```python
from build123d import *

# Parameters (mm, degrees)
HIERRO_ANGULAR_2_X_2_X_0_125_1_DEPTH = 120
CROQUIS3_W                           = 47.625
CROQUIS3_H                           = 45
CORTAR_EXTRUIR1_DEPTH                = 10
CROQUIS4_R                           = 5
CROQUIS4_R_2                         = 2.5
CORTAR_EXTRUIR2_DEPTH                = 10
CROQUIS5_R                           = 16
CORTAR_EXTRUIR3_DEPTH                = 3.175
CROQUIS6_R                           = 2
CORTAR_EXTRUIR4_DEPTH                = 3.175


with BuildPart() as part:
    # Sketch1 → Hierro angular 2 X 2 X 0.125(1) (new body)
    with BuildSketch(Plane(origin=(0, 0, 0), x_dir=(-1, 0, 0), z_dir=(0, 1, 0))):
        with BuildLine():
            Line((0, 0), (0, 50.8))
            Line((0, 50.8), (0.00508, 50.8))
            ThreePointArc((0.00508, 50.8), (2.246551928, 49.871551928), (3.175, 47.63008))
            Line((3.175, 47.63008), (3.175, 7.9375))
            ThreePointArc((3.175, 7.9375), (4.569903955, 4.569903955), (7.9375, 3.175))
            Line((7.9375, 3.175), (47.63008, 3.175))
            ThreePointArc((47.63008, 3.175), (49.871551928, 2.246551928), (50.8, 0.00508))
            Line((50.8, 0.00508), (50.8, 0))
            Line((50.8, 0), (0, 0))
        make_face()
    extrude(amount=HIERRO_ANGULAR_2_X_2_X_0_125_1_DEPTH)

    # Croquis3 → Cortar-Extruir1 (cut)
    with BuildSketch(Plane(origin=(0, 0, 0), x_dir=(-1, 0, 0), z_dir=(0, 0, -1))):
        with Locations((26.9875, 60)):
            Rectangle(CROQUIS3_W, CROQUIS3_H)
    extrude(amount=-CORTAR_EXTRUIR1_DEPTH, mode=Mode.SUBTRACT)

    # Croquis4 → Cortar-Extruir2 (cut)
    with BuildSketch(Plane.ZY.offset(3.175)):
        with Locations((28.175, 12)):
            Circle(CROQUIS4_R)
        with Locations((11.675, 12)):
            Circle(CROQUIS4_R_2)
        with Locations((44.675, 12)):
            Circle(CROQUIS4_R_2)
        with Locations((44.675, 108)):
            Circle(CROQUIS4_R_2)
        with Locations((28.175, 108)):
            Circle(CROQUIS4_R)
        with Locations((11.675, 108)):
            Circle(CROQUIS4_R_2)
    extrude(amount=-CORTAR_EXTRUIR2_DEPTH, mode=Mode.SUBTRACT)

    # Croquis5 → Cortar-Extruir3 (cut)
    with BuildSketch(Plane.ZY.offset(3.175)):
        with Locations((27.63008, 60)):
            Circle(CROQUIS5_R)
    extrude(amount=-CORTAR_EXTRUIR3_DEPTH, mode=Mode.SUBTRACT)

    # Croquis6 → Cortar-Extruir4 (cut)
    with BuildSketch(Plane(origin=(0, 0, 0), x_dir=(-1, 0, 0), z_dir=(0, 0, -1))):
        with Locations((14.175, 35)):
            Circle(CROQUIS6_R)
        with Locations((14.175, 85)):
            Circle(CROQUIS6_R)
        with Locations((44.175, 85)):
            Circle(CROQUIS6_R)
        with Locations((44.175, 35)):
            Circle(CROQUIS6_R)
    extrude(amount=-CORTAR_EXTRUIR4_DEPTH, mode=Mode.SUBTRACT)


solid = part.part
```
Check sheet for the modelled part. Datum: model origin and axes. Units: mm. A direction names the side the tool comes from. Give positions to 0.01 mm unless a question says otherwise; leave off trailing zeros. Order: outer loops, then holes, each group sorted by start corner. A loop starts at its lowest first (then second) coordinate and runs counter-clockwise, first axis right, second up. Notation, with made-up numbers: M 59.5,50.5 L 116.5,50.5 A11 ccw 116.5,56.5 Z; hole C -38,26.5 d1. An arc over 180 degrees is marked long. Answer in a Markdown table with one row per item. Add a question column.
Q1. Sectioned sample at B-B, the plane x = -32. Record the boundary of the cut face in (y, z) (3 decimals).
Q2. Release check for a two-part mould opening along X. For faces 4 (the cylindrical face through (-1.61, 13.502, 32.944)), 5 (the cylindrical face through (-4.53, 100.99, 4.61)), 6 (the cylindrical face through (-13.915, 86.983, 1.565)) record: released by +X, released by -X, zero draft, split by the parting line, or undercut.
Q3. Thickness scan on L1, parallel to X at y = 99, z = 19 (3 decimals); L2, parallel to Z at x = -16, y = 107 (3 decimals); L3, parallel to Y at x = -3, z = 20. Record the ranges inside material, lowest first.
Q4. Sectioned sample at A-A, the plane y = 60. Record the boundary of the cut face in (x, z) (3 decimals).
Q5. Gauge pin test, flat ends, axial feed: pin 1 Ø2.5 at (x, z) = (-31.5, 5) entering from +Y; pin 2 Ø10 at (y, z) = (51, 42) entering from -X (3 decimals); pin 3 Ø5 at (x, y) = (-44.175, 35) entering from -Z; pin 4 Ø2 at (x, y) = (-7.5, 88) entering from +Z. Record the tip position at first contact, or that the pin passes through.
Q6. Access from +Z, -Z, +X, -X, +Y, -Y to the whole of each face (thin tool, end or side, straight path). Record for faces 1 (the flat face through (-27, 37.5, 1)), 2 (the cylindrical face through (-1.61, 110.48, 44.35)), 3 (the flat face through (-28, 101, 3.175)).
Q7. Sectioned sample at C-C, the plane y = 108. Count the separate pieces of the cut face and the enclosed holes in it, and give its area (3 significant figures).
Verdict:
| question | item | result |
|---|---|---|
| 1 | outline | M 0,0 L 37.5,0 L 37.5,3.175 L 0,3.175 Z; M 82.5,0 L 120,0 L 120,3.175 L 82.5,3.175 Z |
| 2 | face 4 | zero draft |
| 2 | face 5 | released by -X |
| 2 | face 6 | undercut |
| 3 | L1 | -3.175 to 0 |
| 3 | L2 | 0 to 3.175 |
| 3 | L3 | 0 to 45.94, 74.06 to 120 |
| 4 | outline | M -3.175,0 L 0,0 L 0,11.63 L -3.175,11.63 Z; M -3.175,43.63 L 0,43.63 L 0,50.8 L -0.005,50.8 A3.17 ccw -3.175,47.63 Z |
| 5 | pin 1 | through |
| 5 | pin 2 | x = -3.175 |
| 5 | pin 3 | z = 0 |
| 5 | pin 4 | z = 3.4 |
| 6 | face 1 | +Z, -Z, -X |
| 6 | face 2 | +X, -X |
| 6 | face 3 | +Z, -X, +Y, -Y |
| 7 | separate pieces | 4 |
| 7 | enclosed holes | 0 |
| 7 | area | 250 mm² |
